Build history of the part. All positions in model axes, mm. A direction names the side the tool comes from. Give positions to 0.01 mm unless a question says otherwise; leave off trailing zeros. Loops run counter-clockwise (first coordinate to the right, second up) from the corner with the lowest first, then second, coordinate; pieces in that order, holes last. Notation, with made-up numbers: M -34,73.5 L 2,73.5 A18 ccw 2,103.5 Z; hole C -10,13 d8. An arc over 180 degrees is marked long. Put each result on its own line as item: value.
```python
from build123d import *

# Parameters (mm, degrees)
SKETCH1_R               = 32.5
SKETCH1_W               = 120.65
SKETCH1_H               = 76.2
BOSS_EXTRUDE2_DEPTH     = 6.35
BOSS_EXTRUDE3_START     = 6.35
SKETCH1_3_R             = 32.5
BOSS_EXTRUDE3_DEPTH     = 19.05
SKETCH2_R               = 3.175
CUT_EXTRUDE1_DEPTH      = 20.05
CUT_EXTRUDE1_DEPTH_BACK = 7.35
SKETCH3_R               = 6.35
CUT_EXTRUDE2_DEPTH      = 19.05
FILLET1_R               = 12.7
SKETCH5_R               = 32.5
BOSS_EXTRUDE6_DEPTH     = 19.05
SKETCH6_R               = 32.5
SKETCH6_R_2             = 27.5
BOSS_EXTRUDE7_DEPTH     = 2.54
SKETCH9_R               = 3.175
CUT_EXTRUDE3_DEPTH      = 1
CUT_EXTRUDE3_DEPTH_BACK = 45.45


with BuildPart() as part:
    # Sketch1 → Boss-Extrude2 (new body)
    with BuildSketch(Plane.XY):
        with BuildLine():
            Line((8.199848, 44.45), (171.45, 44.45))
            Line((171.45, 44.45), (171.45, 38.1))
            Line((171.45, 38.1), (50.8, 38.1))
            Line((50.8, 38.1), (50.8, -38.1))
            Line((50.8, -38.1), (171.45, -38.1))
            Line((171.45, -38.1), (171.45, -44.45))
            Line((171.45, -44.45), (8.199848, -44.45))
            ThreePointArc((8.199848, -44.45), (-45.2, 0), (8.199848, 44.45))
        make_face()
        Circle(SKETCH1_R, mode=Mode.SUBTRACT)
        with Locations((111.125, 0)):
            Rectangle(SKETCH1_W, SKETCH1_H)
    extrude(amount=BOSS_EXTRUDE2_DEPTH)

    # Sketch1<3> → Boss-Extrude3 (add)
    with BuildSketch(Plane.XY.offset(BOSS_EXTRUDE3_START)):
        with BuildLine():
            Line((8.199848, 44.45), (171.45, 44.45))
            Line((171.45, 44.45), (171.45, 38.1))
            Line((171.45, 38.1), (50.8, 38.1))
            Line((50.8, 38.1), (50.8, -38.1))
            Line((50.8, -38.1), (171.45, -38.1))
            Line((171.45, -38.1), (171.45, -44.45))
            Line((171.45, -44.45), (8.199848, -44.45))
            ThreePointArc((8.199848, -44.45), (-45.2, 0), (8.199848, 44.45))
        make_face()
        Circle(SKETCH1_3_R, mode=Mode.SUBTRACT)
    extrude(amount=BOSS_EXTRUDE3_DEPTH)

    # Sketch2 → Cut-Extrude1 (cut, two sides)
    with BuildSketch(Plane.XY.offset(6.35)) as cut_extrude1_sk:
        with Locations((60.325, 28.575)):
            Circle(SKETCH2_R)
        with Locations((161.925, 28.575)):
            Circle(SKETCH2_R)
        with Locations((161.925, -28.575)):
            Circle(SKETCH2_R)
        with Locations((60.325, -28.575)):
            Circle(SKETCH2_R)
    extrude(amount=CUT_EXTRUDE1_DEPTH, mode=Mode.SUBTRACT)
    extrude(cut_extrude1_sk.sketch, amount=-CUT_EXTRUDE1_DEPTH_BACK, mode=Mode.SUBTRACT)

    # Sketch3 → Cut-Extrude2 (cut)
    with BuildSketch(Plane.XY.offset(25.4)):
        with Locations((55.290128, 33.609872)):
            Circle(SKETCH3_R)
        with Locations((55.290128, -33.609872)):
            Circle(SKETCH3_R)
    extrude(amount=-CUT_EXTRUDE2_DEPTH, mode=Mode.SUBTRACT)

    # Fillet1
    fillet1_edges = [part.edges().sort_by_distance(p)[0] for p in [
        (8.199848, -44.45, 12.7),
        (8.199848, 44.45, 12.7),
    ]]
    fillet(fillet1_edges, radius=FILLET1_R)

    # Sketch5 → Boss-Extrude6 (add)
    with BuildSketch(Plane(origin=(0, 0, 0), x_dir=(-1, 0, 0), z_dir=(0, 0, -1))):
        with BuildLine():
            ThreePointArc((-7.2516, -44.614508), (45.2, 0), (-7.2516, 44.614508))
            ThreePointArc((-7.2516, 44.614508), (-45.2, 0), (-7.2516, -44.614508))
        make_face()
        Circle(SKETCH5_R, mode=Mode.SUBTRACT)
    extrude(amount=BOSS_EXTRUDE6_DEPTH)

    # Sketch6 → Boss-Extrude7 (add)
    with BuildSketch(Plane(origin=(0, 0, -19.05), x_dir=(-1, 0, 0), z_dir=(0, 0, -1))):
        Circle(SKETCH6_R)
        Circle(SKETCH6_R_2, mode=Mode.SUBTRACT)
    extrude(amount=-BOSS_EXTRUDE7_DEPTH)

    # Sketch9 → Cut-Extrude3 (cut, two sides)
    with BuildSketch(Plane(origin=(0, 0, -19.05), x_dir=(-1, 0, 0), z_dir=(0, 0, -1))) as cut_extrude3_sk:
        with Locations((36.35, 0)):
            Circle(SKETCH9_R)
        with Locations((18.175, -31.480023)):
            Circle(SKETCH9_R)
        with Locations((-18.175, -31.480023)):
            Circle(SKETCH9_R)
        with Locations((-36.35, 0)):
            Circle(SKETCH9_R)
        with Locations((-18.175, 31.480023)):
            Circle(SKETCH9_R)
        with Locations((18.175, 31.480023)):
            Circle(SKETCH9_R)
    extrude(amount=CUT_EXTRUDE3_DEPTH, mode=Mode.SUBTRACT)
    extrude(cut_extrude3_sk.sketch, amount=-CUT_EXTRUDE3_DEPTH_BACK, mode=Mode.SUBTRACT)


solid = part.part
```
Q1. Mould opens along X. For faces 1 (the cylindrical face through (-34.01, 2.146, 2.864)), 2 (the flat face through (1, -30, -19.05)), 3 (the flat face through (171.45, 1, 4)) say: pulls with the +X half, pulls with the -X half, needs draft (parallel to the pull), parting line crosses it, or undercut.
Here are the results:
face 1: undercut
face 2: needs draft
face 3: pulls with the +X half
Q2. Probe line 1 (X direction, y = 0.5, z = 17.5); line 2 (Y direction, x = 146.5, z = 20); line 3 (Y direction, x = 14.5, z = 6.5). List the from-to ranges inside material, lowest first. Write a range as from..to.
Here are the results:
line 1: -45.2..-39.49, -33.21..-32.5, 32.5..33.21, 39.49..50.8
line 2: -44.45..-38.1, 38.1..44.45
line 3: -44.45..-29.09, 29.09..44.45
Q3. Drop flat-ended pins along their axis: pin 1 Ø3 at (y, z) = (10.5, 13.5) entering from -X; pin 2 Ø15 at (y, z) = (13, 19) entering from +X; pin 3 Ø15 at (x, z) = (122, 17) entering from -Y. Give the stop position or say it passes through.
Here are the results:
pin 1: x = -44.29
pin 2: x = 50.8
pin 3: y = -44.45
Q4. Slice it at A-A (y = 0). List the corners of the cut face in (x, z) (3 decimals), and give its area (3 significant figures).
Here are the results:
outline: M -45.2,-19.05 L -39.525,-19.05 L -39.525,25.4 L -45.2,25.4 Z; M -33.175,-19.05 L -27.5,-19.05 L -27.5,-16.51 L -32.5,-16.51 L -32.5,25.4 L -33.175,25.4 Z; M 27.5,-19.05 L 33.175,-19.05 L 33.175,25.4 L 32.5,25.4 L 32.5,-16.51 L 27.5,-16.51 Z; M 39.525,-19.05 L 45.2,-19.05 L 45.2,0 L 171.45,0 L 171.45,6.35 L 50.8,6.35 L 50.8,25.4 L 39.525,25.4 Z
area: 1,500 mm²
Q5. Slice it at B-B (x = 78). List the corners of the cut face in (y, z).
Here are the results:
outline: M -44.45,0 L 44.45,0 L 44.45,25.4 L 38.1,25.4 L 38.1,6.35 L -38.1,6.35 L -38.1,25.4 L -44.45,25.4 Z
Q6. Tool access for faces 4 (the cylindrical face through (5.961, -26.846, -17.798)), 5 (the flat face through (27, 7, -16.51)), 6 (the flat face through (50.8, 0, 16)), 7 (the flat face through (40, 4, 25.4)), 8 (the flat face through (92, -44.45, 13)): list every direction of +Z, -Z, +X, -X, +Y, -Y with a clear straight run to the whole face (end or side of a thin tool).
Here are the results:
face 4: +Z, -Z
face 5: +Z
face 6: +Z, +X
face 7: +Z, +X, -X, +Y, -Y
face 8: +Z, -Z, +X, -Y
Q7. Slice it at C-C (x = 0). List the corners of the cut face in (y, z), and give its area (3 significant figures).
Here are the results:
outline: M -45.2,-19.05 L -27.5,-19.05 L -27.5,-16.51 L -32.5,-16.51 L -32.5,25.4 L -45.2,25.4 Z; M 27.5,-19.05 L 45.2,-19.05 L 45.2,25.4 L 32.5,25.4 L 32.5,-16.51 L 27.5,-16.51 Z
area: 1,150 mm²
Q8. Slice it at D-D (y = 20). List the corners of the cut face in (x, z), and give its area (3 significant figures).
Here are the results:
outline: M -40.53,-19.05 L -18.87,-19.05 L -18.87,-16.51 L -25.62,-16.51 L -25.62,25.4 L -40.53,25.4 Z; M 18.87,-19.05 L 40.53,-19.05 L 40.53,0 L 171.45,0 L 171.45,6.35 L 50.8,6.35 L 50.8,25.4 L 25.62,25.4 L 25.62,-16.51 L 18.87,-16.51 Z
area: 2,390 mm²
